Geometry: final body of the model. Coordinates: model frame, mm. A direction names the side the tool comes from. Give positions to 0.01 mm unless a question says otherwise; leave off trailing zeros. Write each loop counter-clockwise with the first axis right and the second up, starting at its lowest first coordinate (ties: lowest second). Pieces come first, ordered by that corner, then holes. Notation, with made-up numbers: (70.5, -32) - (118.5, -32) arc R20 ccw to (118.5, -3) - close; hole circle Ø4 at (62.5, -17.75). An arc over 180 degrees is marked (long way). Use CSV: the item, a comma, the result in double quotes. Start each with the question number.
(1) Reachability of faces 4 (the cylindrical face through (-18.03, 1.03, -0.35)), 5 (the cylindrical face through (1.885, 0.583, 1.229)), 6 (the cylindrical face through (0.01, -0.47, 0.23)) from +Z, -Z, +X, -X, +Y, -Y: full face, straight path, thin tool, end or side. Return the list, or none.
(2) Line query: probe 1 along X at (y, z) = (-0.35, 0) (3 decimals); probe 2 along X at (y, z) = (-0.55, -0.35); probe 3 along Z at (x, y) = (-45.5, 0.6). Output: solid intervals per line, ascending. Write a range as [from, to].
(3) Section A-A on x = -44. Output: boundary loops of the cut face in (y, z) (3 decimals).
(4) Section B-B on x = -25. Output: boundary loops of the cut face in (y, z) (3 decimals).
(5) Draft query along X for faces 1 (the flat face through (-0.1, 0.6, 1.575)), 2 (the flat face through (1.3, 0, 0.5)), 3 (the cylindrical face through (2.157, -0.468, -0.465)). Return one class per face: released by +X, released by -X, zero draft, split by the parting line, or undercut.
from build123d import *

# Parameters (mm, degrees)
SKETCH1_W           = 4.5
SKETCH1_H           = 3.15
BOSS_EXTRUDE1_DEPTH = 1.15
BOSS_EXTRUDE2_START = -1.15
SKETCH2_R           = 1.215
SKETCH2_R_2         = 1.05
SKETCH2_R_3         = 0.415
SKETCH2_R_4         = 0.25
BOSS_EXTRUDE2_DEPTH = 2.1
SKETCH3_R           = 0.575
BOSS_EXTRUDE3_DEPTH = 32
SKETCH4_R           = 0.35
BOSS_EXTRUDE4_DEPTH = 32
FILLET1_R           = 1.215
CHAMFER2_SIZE       = 1


with BuildPart() as part:
    # Sketch1 → Boss-Extrude1 (new body)
    with BuildSketch(Plane(origin=(0, 0, 0), x_dir=(1, 0, 0), z_dir=(0, 1, 0))):
        Rectangle(SKETCH1_W, SKETCH1_H)
    extrude(amount=BOSS_EXTRUDE1_DEPTH)

    # Sketch2 → Boss-Extrude2 (add)
    # profile 1 of 2: a face of its own
    with BuildSketch(Plane.XZ.offset(BOSS_EXTRUDE2_START)):
        with Locations((1.035, 0)):
            Circle(SKETCH2_R)
        with Locations(Location((1.035, 0, 0), (0, 0, 270))):
            Circle(SKETCH2_R_2, mode=Mode.SUBTRACT)
    # profile 2 of 2: a face of its own
    with BuildSketch(Plane.XZ.offset(BOSS_EXTRUDE2_START)):
        with Locations(Location((1.035, 0, 0), (0, 0, 270))):
            Circle(SKETCH2_R_3)
        with Locations(Location((1.035, 0, 0), (0, 0, 270))):
            Circle(SKETCH2_R_4, mode=Mode.SUBTRACT)
    extrude(amount=BOSS_EXTRUDE2_DEPTH)

    # Sketch3 → Boss-Extrude3 (add)
    with BuildSketch(Plane.ZY.offset(2.25)):
        with Locations(Location((0, 0.575, 0), (0, 0, 270))):
            Circle(SKETCH3_R)
    extrude(amount=BOSS_EXTRUDE3_DEPTH)

    # Sketch4 → Boss-Extrude4 (add)
    with BuildSketch(Plane.ZY.offset(34.25)):
        with Locations((0, 0.575)):
            Circle(SKETCH4_R)
    extrude(amount=BOSS_EXTRUDE4_DEPTH)

    # Fillet1
    fillet1_edges = [part.edges().sort_by_distance(p)[0] for p in [
        (2.25, 0.575, 1.575),
        (2.25, 0.575, -1.575),
    ]]
    fillet(fillet1_edges, radius=FILLET1_R)

    # Chamfer2
    chamfer2_edges = [part.edges().sort_by_distance(p)[0] for p in [
        (-2.25, 0.575, 1.575),
        (-2.25, 0.575, -1.575),
    ]]
    chamfer(chamfer2_edges, length=CHAMFER2_SIZE - 0.0001)  # a hair under: the kernel refuses the full size


solid = part.part
Check values:
1,face 4,"-X"
1,face 5,"+Z, +X, +Y, -Y"
1,face 6,"-Y"
2,probe 1,"x = [-0.18, -0.015], [0.62, 0.785], [1.285, 1.45], [2.085, 2.25]"
2,probe 2,"x = [-0.13, 0.05], [0.81, 1.26], [2.02, 2.2]"
2,probe 3,"z = [-0.35, 0.35]"
3,outline,"circle Ø0.7 at (0.575, 0)"
4,outline,"circle Ø1.15 at (0.575, 0)"
5,face 1,"zero draft"
5,face 2,"undercut"
5,face 3,"split by the parting line"
